Verification items for this drawing (mm, ordinates from the low corner). Coordinates: 2 decimals unless noted, no trailing zeros. Loops run counter-clockwise (first coordinate to the right, second up) from the corner with the lowest first, then second, coordinate; pieces in that order, holes last. Notation, with made-up numbers: (-24.75, -36.75) - (33.25, -36.75) arc R13 ccw to (33.25, -12.75) - close; hole circle Ø4 at (8.5, 36). An arc over 180 degrees is marked (long way). One line per item, written item: value. Start each with the question number.
(1) Section check B-B (z = 1.1). Count the separate pieces of the cut face and the enclosed holes in it, plus the area to 3 significant figures.
(2) Gauge pin test, flat end, axial feed: P1, Ø3, axis at x = 15, y = 12.5, coming from the -Z side. Record the tip position at first contact, or that the pin passes through.
(3) Thickness scan on probe 1 along Y at (x, z) = (27.5, 1); probe 2 along Y at (x, z) = (45, 1.1); probe 3 along X at (y, z) = (53, 1). Record the ranges inside material, lowest first. Write a range as [from, to].
(4) Section check A-A (y = 53.25). Record the boundary of the cut face in (x, z).
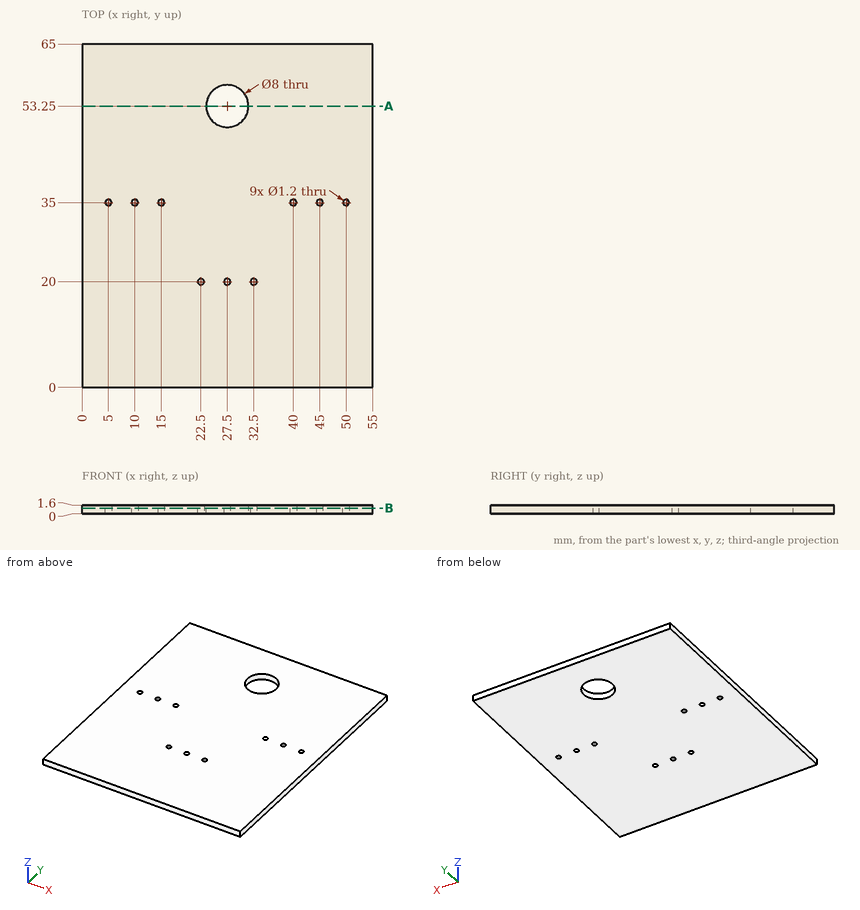
Responses:
1. separate pieces: 1
1. enclosed holes: 10
1. area: 3,510 mm²
2. P1: stops at z = 0
3. probe 1: y = [0, 19.4], [20.6, 49.25], [57.25, 65]
3. probe 2: y = [0, 34.4], [35.6, 65]
3. probe 3: x = [0, 23.51], [31.49, 55]
4. outline: (0, 0) - (23.5, 0) - (23.5, 1.6) - (0, 1.6) - close; (31.5, 0) - (55, 0) - (55, 1.6) - (31.5, 1.6) - close
